Read the model definition and answer for the solid it produces. Units are mm, in the model's axes. Coordinates: 2 decimals unless noted, no trailing zeros. Write each loop counter-clockwise with the first axis right and the second up, starting at its lowest first coordinate (ties: lowest second). Pieces come first, ordered by that corner, then holes.
Item 1: Section A-A (z = -33.05) is taken. Give the vertices of the cut face in (x, y), then the cut area to 3 significant figures.
Item 2: Section B-B (x = 6.5) is taken. Give the vertices of the cut face in (y, z), then the cut area to 4 significant figures.
Item 3: Section C-C (z = -0.05) is taken. Give the vertices of the cut face in (x, y).
Item 4: Straight lines are drawn through the part: probe 1 along X at (y, z) = (1.5, -0.05); probe 2 along Z at (x, y) = (1.5, 1.2); probe 3 along Z at (x, y) = (5, 1.9). For each, find the intervals that lie inside material, in ascending order.
Item 5: Section D-D (y = 0.75) is taken. Give the vertices of the cut face in (x, z).
Item 6: Each of these flat-tipped pins is pushed along its axis until it touches: P1, Ø4.5, axis at x = -23.01, z = -0.05, coming from the +Y side; P2, Ø2, axis at x = 22.99, z = -0.05, coming from the -Y side. Where does it stop, or does it pass through?
from build123d import *

# Parameters (mm, degrees)
SKETCH1_W           = 54.14
SKETCH1_H           = 86.1
BOSS_EXTRUDE1_DEPTH = 2
SKETCH3_R           = 1.8
SKETCH3_W           = 29.974558808
SKETCH3_H           = 36.1
CUT_EXTRUDE1_DEPTH  = 2


with BuildPart() as part:
    # Sketch1 → Boss-Extrude1 (new body)
    with BuildSketch(Plane(origin=(0, 0, 0), x_dir=(1, 0, 0), z_dir=(0, 1, 0))):
        Rectangle(SKETCH1_W, SKETCH1_H)
    extrude(amount=BOSS_EXTRUDE1_DEPTH)

    # Sketch3 → Cut-Extrude1 (cut)
    with BuildSketch(Plane(origin=(0, 2, 0), x_dir=(1, 0, 0), z_dir=(0, 1, 0))):
        with Locations(Location((22.987279404, 0.05, 0), (0, 0, 270))):
            Circle(SKETCH3_R)
        with Locations(Location((-0.012720596, 33.05, 0), (0, 0, 270))):
            Circle(SKETCH3_R)
        with Locations(Location((-0.012720596, -32.95, 0), (0, 0, 270))):
            Circle(SKETCH3_R)
        with Locations(Location((-23.012720596, 0.05, 0), (0, 0, 270))):
            Circle(SKETCH3_R)
        Rectangle(SKETCH3_W, SKETCH3_H)
    extrude(amount=-CUT_EXTRUDE1_DEPTH, mode=Mode.SUBTRACT)


solid = part.part
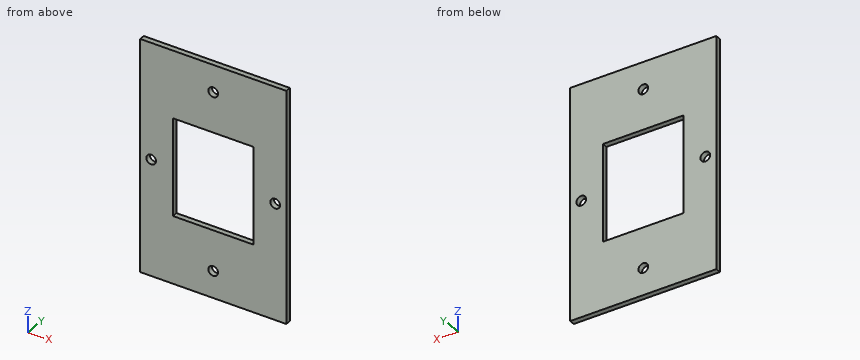
Established:
1. outline: (-27.07, 0) - (-1.81, 0) - (-1.81, 2) - (-27.07, 2) - close; (1.79, 0) - (27.07, 0) - (27.07, 2) - (1.79, 2) - close
1. area: 101 mm2
2. outline: (0, -43.05) - (2, -43.05) - (2, -18.05) - (0, -18.05) - close; (0, 18.05) - (2, 18.05) - (2, 43.05) - (0, 43.05) - close
2. area: 100.0 mm2
3. outline: (-27.07, 0) - (-24.81, 0) - (-24.81, 2) - (-27.07, 2) - close; (-21.21, 0) - (-14.99, 0) - (-14.99, 2) - (-21.21, 2) - close; (14.99, 0) - (21.19, 0) - (21.19, 2) - (14.99, 2) - close; (24.79, 0) - (27.07, 0) - (27.07, 2) - (24.79, 2) - close
4. probe 1: x = -27.07 to -24.81, -21.21 to -14.99, 14.99 to 21.19, 24.79 to 27.07
4. probe 2: z = -43.05 to -34.03, -32.07 to -18.05, 18.05 to 31.97, 33.93 to 43.05
4. probe 3: z = -43.05 to -18.05, 18.05 to 43.05
5. outline: (-27.07, -43.05) - (27.07, -43.05) - (27.07, 43.05) - (-27.07, 43.05) - close; hole circle Ø3.6 at (-23.01, -0.05); hole (-14.99, -18.05) - (14.99, -18.05) - (14.99, 18.05) - (-14.99, 18.05) - close; hole circle Ø3.6 at (-0.01, -33.05); hole circle Ø3.6 at (-0.01, 32.95); hole circle Ø3.6 at (22.99, -0.05)
6. P1: stops at y = 2
6. P2: passes through
